Read the model definition and answer for the solid it produces. Units are mm, in the model's axes. Face numbers are marked on the shaded views. A direction names the side the tool comes from. Round coordinates to 2 decimals unless told otherwise and drop trailing zeros. Write each loop counter-clockwise with the first axis right and the second up, starting at its lowest first coordinate (ties: lowest second). Pieces come first, ordered by that corner, then holes. Notation, with made-up numbers: (-16, -24) - (-1, -24) arc R19 cw to (-1, 3) - close; hole circle Ø1 at (-35.5, 69). An arc over 180 degrees is marked (long way). Use one line per item in the form item = value. Start each with the question number.
1) For the marked faces 4, 5, 6, 7 and 8, determine the directions among +Z, -Z, +X, -X, +Y, -Y from which every point of the face is accessible in a straight line to the end or side of a thin tool.
2) Each of these flat-tipped pins is pushed along its axis until it touches: pin 1 (2 mm diameter, centred on y = 18, z = 8.5, fed in from +X); pin 2 (6 mm diameter, centred on y = 19, z = 5, fed in from -X); pin 3 (0.6 mm diameter, centred on y = 10, z = 8, fed in from -X); pin 4 (5 mm diameter, centred on x = 31.5, y = 2, fed in from +Z). Where does it stop, or does it pass through?
3) The part is cut by section A-A, the plane x = 34. Give the vertices of the cut face in (y, z).
4) For a pull along X with two mould halves and no side action, classify the marked faces 1, 2 and 3 as released by +X, released by -X, zero draft, split by the parting line, or undercut.
5) The part is cut by section B-B, the plane y = 10.5. Give the vertices of the cut face in (x, z), plus the area to 3 significant figures.
6) The part is cut by section D-D, the plane y = 2. Give the vertices of the cut face in (x, z).
7) The part is cut by section C-C, the plane z = -0.5. Give the vertices of the cut face in (x, y), plus the area to 3 significant figures.
8) Consider line 1 along Z through (x, y) = (0, -2); line 2 along X through (y, z) = (20.25, 0); line 3 along X through (y, z) = (6.5, 0.5). Determine where each line is inside the solid, lowest interval first. Write a range as from..to.
from build123d import *

# Parameters (mm, degrees)
SKETCH_1_W               = 80
SKETCH_1_H               = 24
EXTRUDE_1_DEPTH          = 27
EXTRUDE_3_DEPTH          = 24
CUT_EXTRUDE_1_DEPTH      = 54.898051913
CUT_EXTRUDE_3_DEPTH      = 50.729267037
CUT_EXTRUDE_3_DEPTH_BACK = 50.729267037
SKETCH_4_R               = 1.5
CUT_EXTRUDE_4_DEPTH      = 50.729267115
CUT_EXTRUDE_4_DEPTH_BACK = 50.729267115
SKETCH_5_W               = 9
SKETCH_5_H               = 5
SKETCH_6_W               = 9
SKETCH_6_H               = 5
CUT_EXTRUDE_7_DEPTH      = 50.729267115
SKETCH_7_W               = 9
SKETCH_7_H               = 5
CUT_EXTRUDE_8_DEPTH      = 50.729267115
SKETCH_8_W               = 9
SKETCH_8_H               = 5
CUT_EXTRUDE_9_DEPTH      = 50.729267115
SKETCH_9_R               = 2.5
CUT_EXTRUDE_12_DEPTH     = 50.729267115
SKETCH_11_R              = 2.5
CUT_EXTRUDE_13_DEPTH     = 50.729267115
FILLET_1_R               = 3
FILLET_2_R               = 10


with BuildPart() as part:
    # 草图1 → 凸台-拉伸1 (new body)
    with BuildSketch(Plane(origin=(0, 0, 0), x_dir=(1, 0, 0), z_dir=(0, 1, 0))):
        Rectangle(SKETCH_1_W, SKETCH_1_H)
    extrude(amount=EXTRUDE_1_DEPTH)

    # 草图2 → 凸台-拉伸3 (add, through all)
    with BuildSketch(Plane.XY.offset(12)):
        with BuildLine():
            Line((-31, 27), (31, 27))
            ThreePointArc((31, 27), (0, -4), (-31, 27))
        make_face()
    extrude(amount=-EXTRUDE_3_DEPTH)

    # 草图3 → 切除-拉伸1 (cut, through all)
    with BuildSketch(Plane.XY.offset(12)):
        with BuildLine():
            Line((-26, 27), (26, 27))
            ThreePointArc((26, 27), (0, 1), (-26, 27))
        make_face()
    extrude(amount=-CUT_EXTRUDE_1_DEPTH, mode=Mode.SUBTRACT)

    # 草图4 → 切除-拉伸3 (cut, two sides: drawn at the far end of the back side and taken through both)
    with BuildSketch(Plane(origin=(0, 0, 0), x_dir=(1, 0, 0), z_dir=(0, 1, 0)).offset(-CUT_EXTRUDE_3_DEPTH_BACK)):
        with Locations(Location((0, 0, 0), (0, 0, 270))):
            Circle(SKETCH_4_R)
    extrude(amount=CUT_EXTRUDE_3_DEPTH + CUT_EXTRUDE_3_DEPTH_BACK, mode=Mode.SUBTRACT)

    # 草图5 → 切除-拉伸4 (cut, two sides: drawn at the far end of the back side and taken through both)
    with BuildSketch(Plane(origin=(0, 0, 0), x_dir=(1, 0, 0), z_dir=(0, 1, 0)).offset(-CUT_EXTRUDE_4_DEPTH_BACK)):
        with Locations((-35.5, 9.5)):
            Rectangle(SKETCH_5_W, SKETCH_5_H)
    extrude(amount=CUT_EXTRUDE_4_DEPTH + CUT_EXTRUDE_4_DEPTH_BACK, mode=Mode.SUBTRACT)

    # 草图6 → 切除-拉伸7 (cut, through all)
    with BuildSketch(Plane(origin=(0, 0, 0), x_dir=(1, 0, 0), z_dir=(0, 1, 0))):
        with Locations((-35.5, -9.5)):
            Rectangle(SKETCH_6_W, SKETCH_6_H)
    extrude(amount=CUT_EXTRUDE_7_DEPTH, mode=Mode.SUBTRACT)

    # 草图7 → 切除-拉伸8 (cut, through all)
    with BuildSketch(Plane(origin=(0, 0, 0), x_dir=(1, 0, 0), z_dir=(0, 1, 0))):
        with Locations((35.5, 9.5)):
            Rectangle(SKETCH_7_W, SKETCH_7_H)
    extrude(amount=CUT_EXTRUDE_8_DEPTH, mode=Mode.SUBTRACT)

    # 草图8 → 切除-拉伸9 (cut, through all)
    with BuildSketch(Plane(origin=(0, 0, 0), x_dir=(1, 0, 0), z_dir=(0, 1, 0))):
        with Locations((35.5, -9.5)):
            Rectangle(SKETCH_8_W, SKETCH_8_H)
    extrude(amount=CUT_EXTRUDE_9_DEPTH, mode=Mode.SUBTRACT)

    # 草图9 → 切除-拉伸12 (cut, through all)
    with BuildSketch(Plane(origin=(0, 0, 0), x_dir=(1, 0, 0), z_dir=(0, 1, 0))):
        with Locations(Location((-34, 0, 0), (0, 0, 270))):
            Circle(SKETCH_9_R)
    extrude(amount=CUT_EXTRUDE_12_DEPTH, mode=Mode.SUBTRACT)

    # 草图11 → 切除-拉伸13 (cut, through all)
    with BuildSketch(Plane(origin=(0, 0, 0), x_dir=(1, 0, 0), z_dir=(0, 1, 0))):
        with Locations(Location((34, 0, 0), (0, 0, 270))):
            Circle(SKETCH_11_R)
    extrude(amount=CUT_EXTRUDE_13_DEPTH, mode=Mode.SUBTRACT)

    # 圆角1
    fillet_1_edges = [part.edges().sort_by_distance(p)[0] for p in [
        (40, 13.5, 7),
        (31, 13.5, 12),
        (-40, 13.5, -7),
        (-31, 13.5, -12),
        (-40, 13.5, 7),
        (-31, 13.5, 12),
        (40, 13.5, -7),
        (31, 13.5, -12),
    ]]
    fillet(fillet_1_edges, radius=FILLET_1_R)

    # 圆角2
    fillet_2_edges = [part.edges().sort_by_distance(p)[0] for p in [
        (-15.231546212, 0, 0),
        (15.231546212, 0, 0),
    ]]
    fillet(fillet_2_edges, radius=FILLET_2_R)


solid = part.part
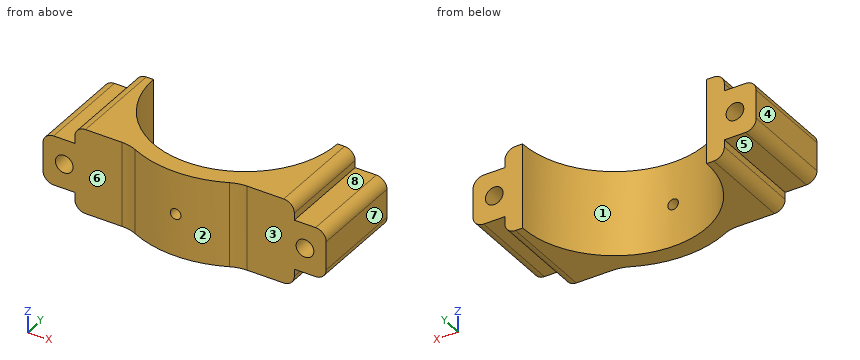
Geometry results:
q1.face_4 = +Z, -Z, -X, +Y, -Y
q1.face_5 = -Z, -X, +Y, -Y
q1.face_6 = +Z, -Z, -X, -Y
q1.face_7 = +Z, -Z, +X, +Y, -Y
q1.face_8 = +Z, +X, +Y, -Y
q2.pin_1 = 31
q2.pin_2 = -40
q2.pin_3 = -31
q2.pin_4 = 11.83
q3.outline = (0, -7) - (27, -7) - (27, -2.5) - (0, -2.5) - close; (0, 2.5) - (27, 2.5) - (27, 7) - (0, 7) - close
q4.face_1 = undercut
q4.face_2 = split by the parting line
q4.face_3 = zero draft
q5.outline = (-40, -4) arc R3 ccw to (-37, -7) - (-31, -7) - (-31, -9) arc R3 ccw to (-28, -12) - (-20.09, -12) - (-20.09, 12) - (-28, 12) arc R3 ccw to (-31, 9) - (-31, 7) - (-37, 7) arc R3 ccw to (-40, 4) - close; (20.09, -12) - (28, -12) arc R3 ccw to (31, -9) - (31, -7) - (37, -7) arc R3 ccw to (40, -4) - (40, 4) arc R3 ccw to (37, 7) - (31, 7) - (31, 9) arc R3 ccw to (28, 12) - (20.09, 12) - close; hole circle Ø5 at (-34, 0); hole circle Ø5 at (34, 0)
q5.area = 721 mm2
q6.outline = (-40, -4) arc R3 ccw to (-37, -7) - (-31, -7) - (-31, -9) arc R3 ccw to (-28, -12) - (-7.14, -12) - (-7.14, 12) - (-28, 12) arc R3 ccw to (-31, 9) - (-31, 7) - (-37, 7) arc R3 ccw to (-40, 4) - close; (7.14, -12) - (28, -12) arc R3 ccw to (31, -9) - (31, -7) - (37, -7) arc R3 ccw to (40, -4) - (40, 4) arc R3 ccw to (37, 7) - (31, 7) - (31, 9) arc R3 ccw to (28, 12) - (7.14, 12) - close; hole circle Ø5 at (-34, 0); hole circle Ø5 at (34, 0)
q7.outline = (-40, 0) - (-36.45, 0) - (-36.45, 27) - (-40, 27) - close; (-31.55, 0) - (-17.66, 0) arc R10 cw to (-13.36, -0.98) arc R31 ccw to (-1.41, -3.97) - (-1.41, 1.04) arc R26 cw to (-26, 27) - (-31.55, 27) - close; (1.41, -3.97) arc R31 ccw to (13.36, -0.98) arc R10 cw to (17.66, 0) - (31.55, 0) - (31.55, 27) - (26, 27) arc R26 cw to (1.41, 1.04) - close; (36.45, 0) - (40, 0) - (40, 27) - (36.45, 27) - close
q7.area = 903 mm2
q8.line_1 = -12..-1.5, 1.5..12
q8.line_2 = -40..-36.5, -31.5..-25.11, 25.11..31.5, 36.5..40
q8.line_3 = -40..-36.45, -31.55..-15.99, 15.99..31.55, 36.45..40
